```python
from build123d import *

# Parameters (mm, degrees)
SKETCH_W     = 38.1
SKETCH_H     = 63.5
PAD_DEPTH    = 2.5
PAD001_DEPTH = 17
SKETCH002_W  = 5
SKETCH002_H  = 15
POCKET_DEPTH = 2.54
PAD002_DEPTH = 20
SKETCH004_W  = 38.1
SKETCH004_H  = 63.5
PAD003_DEPTH = 5


with BuildPart() as part:
    # Sketch → Pad (new body)
    with BuildSketch(Plane.XY):
        with Locations((19.05, 31.75)):
            Rectangle(SKETCH_W, SKETCH_H)
    extrude(amount=PAD_DEPTH)

    # Sketch001 (on Face6 of Pad) → Pad001 (join)
    with BuildSketch(Plane.XY.offset(2.5)):
        Polygon((0, 0), (0, 63.5), (38.1, 63.5), (38.1, 0), (35.56, 0), (35.56, 60.96), (2.54, 60.96), (2.54, 0), align=None)
    extrude(amount=PAD001_DEPTH)

    # Sketch002 (on Face8 of Pad001) → Pocket (cut)
    with BuildSketch(Plane(origin=(0, 0, 0), x_dir=(0, -1, 0), z_dir=(-1, 0, 0))):
        with Locations((-55, 7.5)):
            Rectangle(SKETCH002_W, SKETCH002_H)
    extrude(amount=-POCKET_DEPTH, mode=Mode.SUBTRACT)

    # Sketch003 (on Face9 of Pocket) → Pad002 (join)
    with BuildSketch(Plane.XY.offset(19.5)):
        Polygon((0, 0), (5.55, 0), (5.55, 55.5), (32.55, 55.5), (32.55, 0), (38.1, 0), (38.1, 63.5), (0, 63.5), align=None)
    extrude(amount=PAD002_DEPTH)

    # Sketch004 (on Face12 of Pad002) → Pad003 (join)
    with BuildSketch(Plane.XY.offset(39.5)):
        with Locations((19.05, 31.75)):
            Rectangle(SKETCH004_W, SKETCH004_H)
    extrude(amount=PAD003_DEPTH)


solid = part.part
```
Could you check a few things on this model? Use its own coordinates, in mm. A direction names the side the tool comes from. Round coordinates to 2 decimals unless told otherwise and drop trailing zeros. Loops run counter-clockwise (first coordinate to the right, second up) from the corner with the lowest first, then second, coordinate; pieces in that order, holes last. Notation, with made-up numbers: M 30.25,73 L 50.25,73 A11 ccw 50.25,87 Z; hole C -7,60.25 d10. An arc over 180 degrees is marked long. Answer as CSV lines item,"result".
1) If I drill on probe 1 along X at (y, z) = (38, 36); probe 2 along Z at (x, y) = (30, 57); probe 3 along Z at (x, y) = (17.5, 47.5), over which ranges is the centre line in solid material (lowest first)?
From the geometry:
probe 1,"0 to 5.55, 32.55 to 38.1"
probe 2,"0 to 2.5, 19.5 to 44.5"
probe 3,"0 to 2.5, 39.5 to 44.5"
2) Imagine slicing it at A-A on y = 59. List the corners of the cut face in (x, z) for me.
From the geometry:
outline,"M 0,0 L 38.1,0 L 38.1,44.5 L 0,44.5 Z; hole M 2.54,2.5 L 35.56,2.5 L 35.56,19.5 L 2.54,19.5 Z"
3) For pin 1 Ø4 at (x, z) = (24, 36.5) entering from -Y; pin 2 Ø2 at (x, y) = (1.5, 54) entering from -Z; pin 3 Ø1.2 at (y, z) = (55, 1.5) entering from -X, each with a flat end and sliding along its axis, tell me the tip position at first contact or that it passes through.
From the geometry:
pin 1,"y = 55.5"
pin 2,"z = 15"
pin 3,"x = 2.54"
4) Imagine slicing it at D-D on x = 34. List the corners of the cut face in (y, z) for me.
From the geometry:
outline,"M 0,0 L 63.5,0 L 63.5,44.5 L 0,44.5 L 0,19.5 L 60.96,19.5 L 60.96,2.5 L 0,2.5 Z"
5) Imagine slicing it at C-C on z = 30. List the corners of the cut face in (x, y) for me, and give its area (3 significant figures).
From the geometry:
outline,"M 0,0 L 5.55,0 L 5.55,55.5 L 32.55,55.5 L 32.55,0 L 38.1,0 L 38.1,63.5 L 0,63.5 Z"
area,"921 mm^2"
6) We'd pull the mould along X, two halves only. Please class faces 4 (the flat face through (32.55, 28, 29)), 5 (the flat face through (38.1, 31, 22)), 6 (the flat face through (0, 31, 22)), 7 (the flat face through (36, 0, 22)): released by +X, released by -X, zero draft, split by the parting line, or undercut.
From the geometry:
face 4,"undercut"
face 5,"released by +X"
face 6,"released by -X"
face 7,"zero draft"
7) Which directions (+Z, -Z, +X, -X, +Y, -Y) give clear straight access to the entire face, cutting with the end or side of a thin tool? Please do faces 1 (the flat face through (19, 32, 0)), 2 (the flat face through (1, 52.5, 7)), 3 (the flat face through (19, 28, 39.5)).
From the geometry:
face 1,"-Z, +X, -X, +Y, -Y"
face 2,"-Z, -X"
face 3,"-Y"
8) Imagine slicing it at B-B on z = 5. List the corners of the cut face in (x, y) for me.
From the geometry:
outline,"M 0,0 L 2.54,0 L 2.54,52.5 L 0,52.5 Z; M 0,57.5 L 2.54,57.5 L 2.54,60.96 L 35.56,60.96 L 35.56,0 L 38.1,0 L 38.1,63.5 L 0,63.5 Z"
